The model under review builds one solid part; all positions refer to its coordinate system, in mm. Face numbers are marked on the shaded views. A direction names the side the tool comes from. Give positions to 0.01 mm unless a question says otherwise; leave off trailing zeros. Loops run counter-clockwise (first coordinate to the right, second up) from the corner with the lowest first, then second, coordinate; pieces in that order, holes last. Notation, with made-up numbers: M 46.25,-8 L 97.25,-8 A22 cw 97.25,19 Z; hole C -26,35.5 d1. An arc over 180 degrees is marked long. Return JSON: item names as keys, results as strings.
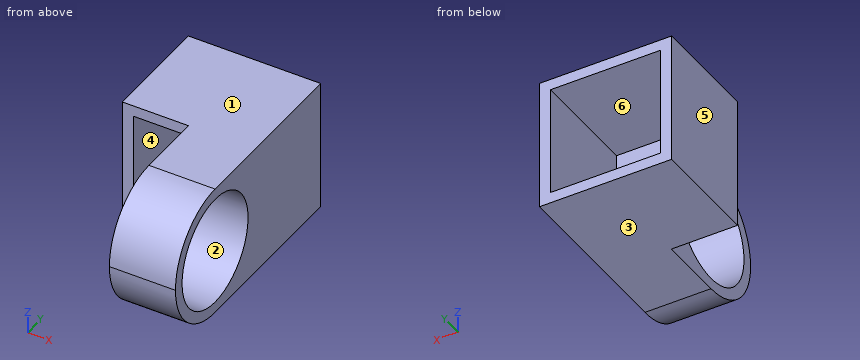
```python
from build123d import *

# Parameters (mm, degrees)
SKETCH_1_W          = 12
SKETCH_1_H          = 12
SKETCH_1_W_2        = 10
SKETCH_1_H_2        = 10
EXTRUDE_1_DEPTH     = 10
EXTRUDE_2_DEPTH     = 6
SKETCH_4_R          = 5
CUT_EXTRUDE_1_DEPTH = 6


with BuildPart() as part:
    # 草图1 → 凸台-拉伸1 (new body)
    with BuildSketch(Plane(origin=(0, 0, 0), x_dir=(1, 0, 0), z_dir=(0, 1, 0))):
        Rectangle(SKETCH_1_W, SKETCH_1_H)
        Rectangle(SKETCH_1_W_2, SKETCH_1_H_2, mode=Mode.SUBTRACT)
    extrude(amount=EXTRUDE_1_DEPTH)

    # 草图3 → 凸台-拉伸2 (add)
    with BuildSketch(Plane(origin=(6, 0, 0), x_dir=(0, 0, -1), z_dir=(1, 0, 0))):
        Polygon((0, -6), (-6, 0), (-6, -6), align=None)
        Polygon((6, 0), (-6, 0), (0, -6), (6, -6), align=None)
        with BuildLine():
            Line((0, -6), (-6, -6))
            ThreePointArc((-6, -6), (-4.242640687, -10.242640687), (0, -12))
            ThreePointArc((0, -12), (2.296100594, -11.543277195), (4.242640687, -10.242640687))
            Line((4.242640687, -10.242640687), (0, -6))
        make_face()
        with BuildLine():
            Line((6, -6), (0, -6))
            Line((0, -6), (4.242640687, -10.242640687))
            ThreePointArc((4.242640687, -10.242640687), (5.543277195, -8.296100594), (6, -6))
        make_face()
    extrude(amount=-EXTRUDE_2_DEPTH)

    # 草图4 → 切除-拉伸1 (cut)
    with BuildSketch(Plane(origin=(6, 0, 0), x_dir=(0, 0, -1), z_dir=(1, 0, 0))):
        with Locations((0, -6)):
            Circle(SKETCH_4_R)
    extrude(amount=-CUT_EXTRUDE_1_DEPTH, mode=Mode.SUBTRACT)


solid = part.part
```
1) Consider section B-B on y = 1.25. Write out the cut boundary in (x, z).
From the geometry:
{"outline": "M -6,-6 L 6,-6 L 6,6 L -6,6 Z; hole M -5,-5 L 5,-5 L 5,5 L -5,5 Z"}
2) Consider section C-C on z = -0.5. Write out the cut boundary in (x, y), then the cut area to 3 significant figures.
From the geometry:
{"outline": "M -6,0 L -5,0 L -5,10 L -6,10 Z; M 0,-11.98 L 6,-11.98 L 6,-10.97 L 0,-10.97 Z; M 0,-1.03 L 6,-1.03 L 6,10 L 5,10 L 5,0 L 0,0 Z", "area": "32.2 mm²"}
3) The part is to be moulded in two halves that separate along Z. For the marked faces 1, 2, 3 and 4, say which applies: released by +Z, released by -Z, zero draft, split by the parting line, or undercut.
From the geometry:
{"face 1": "released by +Z", "face 2": "undercut", "face 3": "released by -Z", "face 4": "undercut"}
4) Insertion check: pin 1 (3.5 mm diameter, centred on y = -4, z = -1.5, fed in from -X); pin 2 (1.8 mm diameter, centred on x = -4.5, z = 2, fed in from -Y). Each pin has a flat end and moves straight along its axis. Give the tip position at first contact, or say it passes through.
From the geometry:
{"pin 1": "through", "pin 2": "y = 0"}
5) Tool access review of the marked faces 5 and 6: name each direction out of +Z, -Z, +X, -X, +Y, -Y from which nothing blocks a thin tool from reaching the whole face with its end or side.
From the geometry:
{"face 5": "+Z, -Z, -X, +Y, -Y", "face 6": "+Y"}
6) Wall thickness on L1, parallel to X at y = 1.75, z = -3.25; L2, parallel to Y at x = 2.45, z = 0: over which ranges is each line inside the solid? List them lowest first. Write a range as from..to.
From the geometry:
{"L1": "-6..-5, 5..6", "L2": "-12..-11, -1..0"}
7) Consider section D-D on z = -2. Write out the cut boundary in (x, y).
From the geometry:
{"outline": "M -6,0 L -5,0 L -5,10 L -6,10 Z; M 0,-11.66 L 6,-11.66 L 6,-10.58 L 0,-10.58 Z; M 0,-1.42 L 6,-1.42 L 6,10 L 5,10 L 5,0 L 0,0 Z"}
8) Consider section A-A on x = -1.25. Write out the cut boundary in (y, z), then the cut area to 3 significant figures.
From the geometry:
{"outline": "M 0,-6 L 10,-6 L 10,-5 L 0,-5 Z; M 0,5 L 10,5 L 10,6 L 0,6 Z", "area": "20.0 mm²"}
